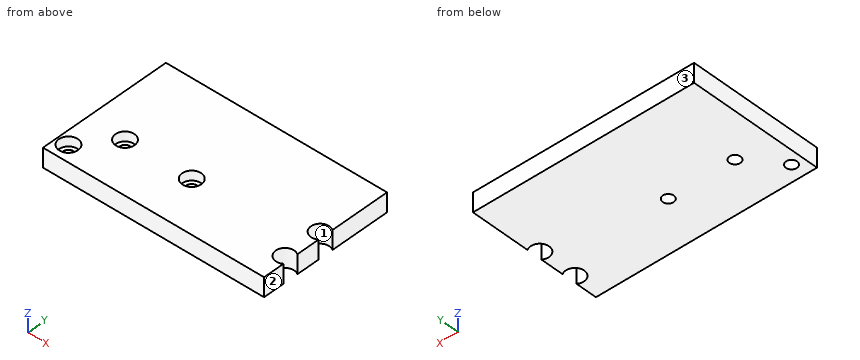
```python
from build123d import *

# Parameters (mm, degrees)
SKETCH_1_W                   = 116
SKETCH_1_H                   = 70
EXTRUDE_1_DEPTH              = 10
SKETCH_2_R                   = 4.85
CUT_EXTRUDE_1_DEPTH          = 136.852861582
HOLE_WIZARD_M5_1_D           = 5.8
HOLE_WIZARD_M5_1_CBORE_D     = 10
HOLE_WIZARD_M5_1_CBORE_DEPTH = 5


with BuildPart() as part:
    # 草图1 → 凸台-拉伸1 (new body)
    with BuildSketch(Plane.XY):
        with Locations((58, 35)):
            Rectangle(SKETCH_1_W, SKETCH_1_H)
    extrude(amount=EXTRUDE_1_DEPTH)

    # 草图2 → 切除-拉伸1 (cut, through all)
    with BuildSketch(Plane.XY.offset(10)):
        with Locations((113.2, 35)):
            Circle(SKETCH_2_R)
        with Locations((113.2, 15)):
            Circle(SKETCH_2_R)
    extrude(amount=-CUT_EXTRUDE_1_DEPTH, mode=Mode.SUBTRACT)

    # M5 六角凹头螺钉的柱形沉头孔1 (through all)
    with Locations(Plane.XY.offset(10)):
        with Locations((6, 8), (20, 25), (55, 25)):
            CounterBoreHole(HOLE_WIZARD_M5_1_D / 2, HOLE_WIZARD_M5_1_CBORE_D / 2, HOLE_WIZARD_M5_1_CBORE_DEPTH)


solid = part.part
```
Build history of the part. All positions in model axes, mm. Face numbers are marked on the shaded views. Coordinates: 2 decimals unless noted, no trailing zeros. Write each loop counter-clockwise with the first axis right and the second up, starting at its lowest first coordinate (ties: lowest second). Pieces come first, ordered by that corner, then holes.
1. Band-saw the part on C-C, the plane z = 2.25. Give the cut face in (x, y).
Answer block:
outline: (0, 0) - (116, 0) - (116, 11.04) arc R4.85 cw (long way) to (116, 18.96) - (116, 31.04) arc R4.85 cw (long way) to (116, 38.96) - (116, 70) - (0, 70) - close; hole circle Ø5.8 at (6, 8); hole circle Ø5.8 at (20, 25); hole circle Ø5.8 at (55, 25)
2. Band-saw the part on A-A, the plane y = 25. Give the cut face in (x, z), and give its area (3 significant figures).
Answer block:
outline: (0, 0) - (17.1, 0) - (17.1, 5) - (15, 5) - (15, 10) - (0, 10) - close; (22.9, 0) - (52.1, 0) - (52.1, 5) - (50, 5) - (50, 10) - (25, 10) - (25, 5) - (22.9, 5) - close; (57.9, 0) - (116, 0) - (116, 10) - (60, 10) - (60, 5) - (57.9, 5) - close
area: 1,000 mm2
3. Band-saw the part on D-D, the plane y = 8. Give the cut face in (x, z), and give its area (3 significant figures).
Answer block:
outline: (0, 0) - (3.1, 0) - (3.1, 5) - (1, 5) - (1, 10) - (0, 10) - close; (8.9, 0) - (116, 0) - (116, 10) - (11, 10) - (11, 5) - (8.9, 5) - close
area: 1,080 mm2
4. Band-saw the part on B-B, the plane x = 6. Give the cut face in (y, z).
Answer block:
outline: (0, 0) - (5.1, 0) - (5.1, 5) - (3, 5) - (3, 10) - (0, 10) - close; (10.9, 0) - (70, 0) - (70, 10) - (13, 10) - (13, 5) - (10.9, 5) - close
5. Drill centre lines: probe 1 along X at (y, z) = (27.5, 6.75); probe 2 along Y at (x, z) = (20, 7.7); probe 3 along Y at (x, z) = (55, 3.5). Where is each one in solid material? Low to high.
Answer block:
probe 1: x = 0 to 15.67, 24.33 to 50.67, 59.33 to 116
probe 2: y = 0 to 20, 30 to 70
probe 3: y = 0 to 22.1, 27.9 to 70
6. Pull direction Y, two halves, no side cores. Call the marked faces 1, 2 and 3: released by +Y, released by -Y, zero draft, split by the parting line, or undercut.
Answer block:
face 1: undercut
face 2: zero draft
face 3: released by +Y
7. Drop flat-ended pins along their axis: pin 1 (1 mm diameter, centred on y = 41.5, z = 4, fed in from -X); pin 2 (3 mm diameter, centred on x = 54.5, y = 23.5, fed in from +Z); pin 3 (3.5 mm diameter, centred on x = 55, y = 25, fed in from -Z). Give the stop position or say it passes through.
Answer block:
pin 1: stops at x = 0
pin 2: stops at z = 5
pin 3: passes through
